Input: part model. Units: mm. Frame: model coordinates. A direction names the side the tool comes from. Coordinates: 2 decimals unless noted, no trailing zeros. Loops run counter-clockwise (first coordinate to the right, second up) from the corner with the lowest first, then second, coordinate; pieces in that order, holes last. Notation, with made-up numbers: (76, 19) -> (100, 19) arc R29 ccw to (100, 45) -> close; hole circle Ø5 at (-13.5, -5). An arc over 180 degrees is marked (long way). Put each result on its own line as item: value. Start each with the question number.
1) Cut plane B-B (z = -20). Return the cut outline in (x, y), plus the area to 3 significant figures.
2) Set-up query: faces 1 (the flat face through (-31, -98.298, 96)), 2 (the flat face through (-27.76, -96.69, 72.62)). Return all of +Z, -Z, +X, -X, +Y, -Y with unobstructed straight access to the full face (end or side cutting, diameter ignored); none if empty.
3) Cut plane A-A (x = 0). Return the cut outline in (y, z) (1 decimal), plus the area to 3 significant figures.
4) Pull-direction query (X, two-part tool) for faces 3 (the cylindrical face through (-9.57, -96.688, 74.888)), 4 (the flat face through (115, 6.984, -23)), 5 (the cylindrical face through (-70.2, -96.7, 68.5)); classes: pulls with the +X half, pulls with the -X half, needs draft (parallel to the pull), parting line crosses it, or undercut.
5) Material intervals for L1, parallel to X at y = -46, z = -68.5; L2, parallel to X at y = -9.5, z = 107; L3, parallel to Z at x = 0, y = -65.5 (1 decimal), sorted ascending.
6) Cut plane C-C (y = -48.5). Return the cut outline in (x, z) (3 decimals), plus the area to 3 significant figures.
7) Cut plane D-D (x = -78). Return the cut outline in (y, z).
8) Contact query for flat-ended pins moving along their axis: P1, Ø2.5, axis at x = 119, y = -28.5, coming from the +Z side; P2, Ø3, axis at x = 15, y = -28.5, coming from the -Z side; P3, Ø12, axis at y = -42, z = -13, coming from the +X side; P4, Ø6.5, axis at x = -10.62, z = 78.23, coming from the -Y side. Output: stop coordinate, or through.
from build123d import *

# Parameters (mm, degrees)
BASE_FLANGE1_DEPTH  = 98.298
CUT_EXTRUDE1_START  = -19.939
CUT_EXTRUDE1_DEPTH  = 19.939
BOSS_EXTRUDE3_START = -3.175
SKETCH13_R          = 3.5
BOSS_EXTRUDE3_DEPTH = 3.175
BOSS_EXTRUDE4_START = 4.572
BOSS_EXTRUDE4_DEPTH = 4.572
BOSS_EXTRUDE5_START = 2.4115014
BOSS_EXTRUDE5_DEPTH = 2.4115014


# Sheet-metal steps are written as plain solids
with BuildPart() as part:
    # Sketch3 → Base-Flange1 (new body)
    with BuildSketch(Plane(origin=(0, 0, 0), x_dir=(1, 0, 0), z_dir=(0, 1, 0))):
        with BuildLine():
            Line((116.647348933, 2.54), (119.822348933, 2.54))
            ThreePointArc((119.822348933, 2.54), (-109.127582861, 50.474671088), (75.651891683, -92.955973295))
            Line((75.651891683, -92.955973295), (73.645289253, -90.495452836))
            ThreePointArc((73.645289253, -90.495452836), (-105.909021844, 48.952371802), (116.647348933, 2.54))
        make_face()
    extrude(amount=-BASE_FLANGE1_DEPTH)

    # Sketch11 → Cut-Extrude1 (cut)
    with BuildSketch(Plane.XZ.offset(98.298).offset(CUT_EXTRUDE1_START)):
        with BuildLine():
            Line((32.000435674, 115.55214828), (29.730194096, 112.823628607))
            ThreePointArc((29.730194096, 112.823628607), (52.879669985, 104.003827407), (73.645289253, 90.495452836))
            Line((73.645289253, 90.495452836), (75.651891683, 92.955973295))
            ThreePointArc((75.651891683, 92.955973295), (54.995189309, 106.512393046), (32.000435674, 115.55214828))
        make_face()
        with BuildLine():
            Line((-92.337333522, 76.828501251), (-89.68916988, 74.625119225))
            ThreePointArc((-89.68916988, 74.625119225), (-40.869300957, -109.282916562), (116.647348933, -2.54))
            Line((116.647348933, -2.54), (119.822348933, -2.54))
            ThreePointArc((119.822348933, -2.54), (-42.24188113, -112.507437016), (-92.337333522, 76.828501251))
        make_face()
    extrude(amount=CUT_EXTRUDE1_DEPTH, mode=Mode.SUBTRACT)

    # Sketch13 → Boss-Extrude3 (add)
    with BuildSketch(Plane.XZ.offset(98.298).offset(BOSS_EXTRUDE3_START)):
        with BuildLine():
            Line((-37.903446615, 31.537248793), (29.730194096, 112.823628607))
            ThreePointArc((29.730194096, 112.823628607), (-35.546465704, 111.128323973), (-89.68916988, 74.625119225))
            Line((-89.68916988, 74.625119225), (-37.903446615, 31.537248793))
        make_face()
        with Locations(Location((-10.621108202, 78.226237974, 0), (0, 0, 270))):
            Circle(SKETCH13_R, mode=Mode.SUBTRACT)
        with Locations(Location((10.39338393, 103.482781479, 0), (0, 0, 270))):
            Circle(SKETCH13_R, mode=Mode.SUBTRACT)
        with BuildLine():
            Line((-53.950312206, 61.001291051), (-21.551148637, 99.940651521))
            ThreePointArc((-21.551148637, 99.940651521), (-12.608395426, 100.76050822), (-11.788538727, 91.817755009))
            Line((-11.788538727, 91.817755009), (-44.187702296, 52.878394539))
            ThreePointArc((-44.187702296, 52.878394539), (-53.130455507, 52.05853784), (-53.950312206, 61.001291051))
        make_face(mode=Mode.SUBTRACT)
        with BuildLine():
            Line((-71.024350753, 77.519358691), (-51.203588088, 100.902170675))
            ThreePointArc((-51.203588088, 100.902170675), (-42.25369967, 101.640071282), (-41.515799064, 92.690182864))
            Line((-41.515799064, 92.690182864), (-61.336561728, 69.30737088))
            ThreePointArc((-61.336561728, 69.30737088), (-70.286450146, 68.569470273), (-71.024350753, 77.519358691))
        make_face(mode=Mode.SUBTRACT)
    extrude(amount=BOSS_EXTRUDE3_DEPTH)

    # Sketch14 → Boss-Extrude4 (add)
    with BuildSketch(Plane(origin=(0, 0, 0), x_dir=(1, 0, 0), z_dir=(0, 1, 0)).offset(BOSS_EXTRUDE4_START)):
        with BuildLine():
            Line((116.647348933, 2.54), (119.822348933, 2.54))
            ThreePointArc((119.822348933, 2.54), (-109.127582861, 50.474671088), (75.651891683, -92.955973295))
            Line((75.651891683, -92.955973295), (73.645289253, -90.495452836))
            ThreePointArc((73.645289253, -90.495452836), (-105.909021844, 48.952371802), (116.647348933, 2.54))
        make_face()
    extrude(amount=-BOSS_EXTRUDE4_DEPTH)

    # Sketch15 → Boss-Extrude5 (add)
    with BuildSketch(Plane(origin=(0, 4.572, 0), x_dir=(1, 0, 0), z_dir=(0, 1, 0)).offset(BOSS_EXTRUDE5_START)):
        with BuildLine():
            Line((116.647348933, 2.54), (119.822348933, 2.54))
            ThreePointArc((119.822348933, 2.54), (117.525772125, 23.578469398), (111.569940957, 43.886584395))
            Line((111.569940957, 43.886584395), (108.304935184, 43.394661284))
            ThreePointArc((108.304935184, 43.394661284), (114.316045984, 23.343034156), (116.647348933, 2.54))
        make_face()
    extrude(amount=-BOSS_EXTRUDE5_DEPTH)


solid = part.part
Results found:
1. outline: (-118.55, -78.36) -> (-114.95, -78.36) -> (-114.95, 4.57) -> (-118.55, 4.57) -> close; (114.95, -78.36) -> (118.18, -78.36) -> (118.18, 6.98) -> (114.95, 6.98) -> close
1. area: 575 mm2
2. face 1: +Z, -Z, +X, -X, -Y
2. face 2: +Y, -Y
3. outline: (-98.3, 77.1) -> (-95.1, 77.1) -> (-95.1, 116.7) -> (4.6, 116.7) -> (4.6, 119.9) -> (-98.3, 119.9) -> close; (-78.4, -120.1) -> (4.6, -120.1) -> (4.6, -116.7) -> (-78.4, -116.7) -> close
3. area: 748 mm2
4. face 3: undercut
4. face 4: needs draft
4. face 5: undercut
5. L1: x = -98.81 to -94.45, 94.45 to 98.44
5. L2: x = -54.41 to -46.52, 46.52 to 54.04
5. L3: z = -120.1 to -116.7, 116.7 to 119.9
6. outline: (73.645, 90.495) -> (75.652, 92.956) arc R120.032 ccw (long way) to (119.822, -2.54) -> (116.647, -2.54) arc R116.675 cw (long way) to start
6. area: 2,160 mm2
7. outline: (-98.3, 64.9) -> (-95.12, 64.9) -> (-95.12, 86.77) -> (4.57, 86.77) -> (4.57, 91.31) -> (-98.3, 91.31) -> close; (-78.36, -91.48) -> (4.57, -91.48) -> (4.57, -86.77) -> (-78.36, -86.77) -> close
8. P1: stops at z = -2.54
8. P2: stops at z = -119.33
8. P3: stops at x = 119.65
8. P4: passes through
